```python
from build123d import *

# Parameters (mm, degrees)
SKETCH_1_W          = 20
SKETCH_1_H          = 19
SKETCH_1_R          = 3
EXTRUDE_1_DEPTH     = 18
SKETCH_1_H_2        = 20
EXTRUDE_1_2_DEPTH   = 18
SKETCH_2_W          = 20
SKETCH_2_H          = 109
SKETCH_2_R          = 3
EXTRUDE_2_DEPTH     = 4
EXTRUDE_3_DEPTH     = 6
SKETCH_4_R          = 0.9
CUT_EXTRUDE_1_DEPTH = 788.391009845
SKETCH_5_R          = 3
EXTRUDE_4_DEPTH     = 13
CHAMFER_1_SIZE      = 2
SKETCH_6_W          = 3.5
SKETCH_6_H          = 12.5
EXTRUDE_5_DEPTH     = 5
FILLET_1_R          = 4
CHAMFER_2_SIZE      = 2


with BuildPart() as part:
    # Sketch 1 → Extrude 1 (new body)
    with BuildSketch(Plane(origin=(0, 0, 241.9894311), x_dir=(-1, 0, 0), z_dir=(0, 0, -1))):
        with Locations((770.850538245, -0.64131648)):
            Rectangle(SKETCH_1_W, SKETCH_1_H)
        with Locations(Location((770.850538245, -1.14131648, 0), (0, 0, 90))):
            Circle(SKETCH_1_R, mode=Mode.SUBTRACT)
    extrude(amount=EXTRUDE_1_DEPTH)



with BuildPart() as body_2:
    # Sketch 1 → Extrude 1 2 (new body)
    with BuildSketch(Plane(origin=(0, 0, 241.9894311), x_dir=(-1, 0, 0), z_dir=(0, 0, -1))):
        with Locations((770.850538245, 88.85868352)):
            Rectangle(SKETCH_1_W, SKETCH_1_H_2)
        with Locations(Location((770.850538245, 88.85868352, 0), (0, 0, 90))):
            Circle(SKETCH_1_R, mode=Mode.SUBTRACT)
    extrude(amount=EXTRUDE_1_2_DEPTH)


with BuildPart() as part_1:
    add(part.part)

    add(body_2.part)  # Extrude 2 merges body 2
    # Sketch 2 → Extrude 2 (add)
    with BuildSketch(Plane(origin=(0, 0, 223.9894311), x_dir=(-1, 0, 0), z_dir=(0, 0, -1))):
        with Locations((770.850538245, 44.35868352)):
            Rectangle(SKETCH_2_W, SKETCH_2_H)
        with Locations(Location((770.850538245, 88.85868352, 0), (0, 0, 90))):
            Circle(SKETCH_2_R, mode=Mode.SUBTRACT)
        with Locations(Location((770.850538245, -1.14131648, 0), (0, 0, 90))):
            Circle(SKETCH_2_R, mode=Mode.SUBTRACT)
    extrude(amount=EXTRUDE_2_DEPTH)

    # Sketch 3 → Extrude 3 (add)
    with BuildSketch(Plane(origin=(0, 0, 219.9894311), x_dir=(-1, 0, 0), z_dir=(0, 0, -1))):
        Polygon((780.850538245, 59.85868352), (780.850538245, 51.85868352), (777.850538245, 51.85868352), (777.850538245, 48.60868352), (769.850538245, 48.60868352), (769.850538245, 61.10868352), (777.850538245, 61.10868352), (777.850538245, 59.85868352), align=None)
    extrude(amount=EXTRUDE_3_DEPTH)

    # Sketch 4 → Cut-Extrude 1 (cut, through all)
    with BuildSketch(Plane(origin=(0, 0, 219.9894311), x_dir=(-1, 0, 0), z_dir=(0, 0, -1))):
        with Locations(Location((775.850538245, 50.85868352, 0), (0, 0, 90))):
            Circle(SKETCH_4_R)
        with Locations(Location((775.850538245, 58.85868352, 0), (0, 0, 90))):
            Circle(SKETCH_4_R)
    extrude(amount=CUT_EXTRUDE_1_DEPTH, mode=Mode.SUBTRACT)

    # Sketch 5 → Extrude 4 (add)
    # profile 1 of 2: a face of its own
    with BuildSketch(Plane(origin=(0, 0, 219.9894311), x_dir=(-1, 0, 0), z_dir=(0, 0, -1))):
        Polygon((760.850538245, -10.14131648), (780.850538245, -10.14131648), (780.850538245, 51.85868352), (777.850538245, 51.85868352), (777.850538245, 48.60868352), (760.850538245, 48.60868352), align=None)
        with Locations(Location((770.850538245, -1.14131648, 0), (0, 0, 90))):
            Circle(SKETCH_5_R, mode=Mode.SUBTRACT)
    # profile 2 of 2: a face of its own
    with BuildSketch(Plane(origin=(0, 0, 219.9894311), x_dir=(-1, 0, 0), z_dir=(0, 0, -1))):
        Polygon((777.850538245, 61.10868352), (777.850538245, 59.85868352), (780.850538245, 59.85868352), (780.850538245, 98.85868352), (760.850538245, 98.85868352), (760.850538245, 61.10868352), align=None)
        with Locations(Location((770.850538245, 88.85868352, 0), (0, 0, 90))):
            Circle(SKETCH_5_R, mode=Mode.SUBTRACT)
    extrude(amount=EXTRUDE_4_DEPTH)

    # Chamfer 1
    chamfer_1_edges = [part_1.edges().sort_by_distance(p)[0] for p in [
        (-780.850538245, 59.85868352, 210.4894311),
        (-780.850538245, 55.85868352, 213.9894311),
        (-780.850538245, 51.85868352, 210.4894311),
    ]]
    chamfer(chamfer_1_edges, length=CHAMFER_1_SIZE)

    # Sketch 6 → Extrude 5 (add)
    with BuildSketch(Plane(origin=(0, 0, 206.9894311), x_dir=(-1, 0, 0), z_dir=(0, 0, -1))):
        with Locations((762.600538245, 54.85868352)):
            Rectangle(SKETCH_6_W, SKETCH_6_H)
    extrude(amount=-EXTRUDE_5_DEPTH)

    # Fillet 1
    fillet_1_edges = [part_1.edges().sort_by_distance(p)[0] for p in [
        (-780.850538245, 98.85868352, 224.4894311),
        (-780.850538245, 78.85868352, 232.9894311),
        (-780.850538245, 8.85868352, 232.9894311),
        (-780.850538245, -10.14131648, 224.4894311),
    ]]
    fillet(fillet_1_edges, radius=FILLET_1_R)

    # Chamfer 2
    chamfer_2_edges = [part_1.edges().sort_by_distance(p)[0] for p in [
        (-760.850538245, 98.85868352, 224.4894311),
        (-760.850538245, -10.14131648, 224.4894311),
    ]]
    chamfer(chamfer_2_edges, length=CHAMFER_2_SIZE)


solid = part_1.part
```
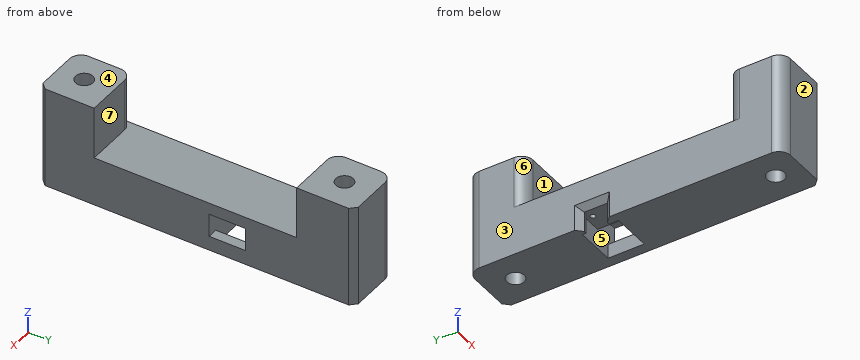
Build history of the part. All positions in model axes, mm. Face numbers are marked on the shaded views. A direction names the side the tool comes from. Coordinates: 2 decimals unless noted, no trailing zeros. Order: outer loops, then holes, each group sorted by start corner. A loop starts at its lowest first (then second) coordinate and runs counter-clockwise, first axis right, second up.
Item 1: Drop flat-ended pins along their axis: pin 1 Ø2 at (x, y) = (-776, 50.5) entering from -Z; pin 2 Ø1.1 at (x, z) = (-778.5, 210.5) entering from +Y; pin 3 Ø10 at (x, y) = (-772.5, 52) entering from +Z; pin 4 Ø5 at (x, y) = (-770.85, 88.86) entering from -Z. Give the stop position or say it passes through.
Filled in:
pin 1: stops at z = 213.99
pin 2: stops at y = 98.7
pin 3: stops at z = 223.99
pin 4: passes through
Item 2: Saw through at D-D on z = 215. List the corners of the cut face in (x, y), then the cut area to 3 significant figures.
Filled in:
outline: (-780.85, -6.14) arc R4 ccw to (-776.85, -10.14) - (-762.85, -10.14) - (-760.85, -8.14) - (-760.85, 48.61) - (-769.85, 48.61) - (-769.85, 61.11) - (-760.85, 61.11) - (-760.85, 96.86) - (-762.85, 98.86) - (-776.85, 98.86) arc R4 ccw to (-780.85, 94.86) - (-780.85, 61.86) - (-779.86, 60.87) - (-779.86, 50.85) - (-780.85, 49.86) - close; hole circle Ø1.8 at (-775.85, 50.86); hole circle Ø1.8 at (-775.85, 58.86); hole circle Ø6 at (-770.85, -1.14); hole circle Ø6 at (-770.85, 88.86)
area: 1,980 mm2
Item 3: Saw through at A-A on y = 55. List the corners of the cut face in (x, z), then the cut area to 4 significant figures.
Filled in:
outline: (-780.85, 215.99) - (-778.85, 213.99) - (-769.85, 213.99) - (-769.85, 219.99) - (-760.85, 219.99) - (-760.85, 223.99) - (-780.85, 223.99) - close; (-764.35, 206.99) - (-760.85, 206.99) - (-760.85, 211.99) - (-764.35, 211.99) - close
area: 161.5 mm2
Item 4: Mould opens along Y. For the marked faces 1, 2 and 3 say: released by +Y, released by -Y, zero draft, split by the parting line, or undercut.
Filled in:
face 1: undercut
face 2: released by -Y
face 3: zero draft
Item 5: Saw through at C-C on x = -772. List the corners of the cut face in (y, z), then the cut area to 3 significant figures.
Filled in:
outline: (-10.14, 206.99) - (-3.91, 206.99) - (-3.91, 241.99) - (-10.14, 241.99) - close; (1.63, 206.99) - (48.61, 206.99) - (48.61, 213.99) - (61.11, 213.99) - (61.11, 206.99) - (86.09, 206.99) - (86.09, 241.99) - (78.86, 241.99) - (78.86, 223.99) - (8.86, 223.99) - (8.86, 241.99) - (1.63, 241.99) - close; (91.63, 206.99) - (98.86, 206.99) - (98.86, 241.99) - (91.63, 241.99) - close
area: 2,080 mm2
Item 6: Tool access for the marked faces 4, 5, 6 and 7: list every direction of +Z, -Z, +X, -X, +Y, -Y with a clear straight run to the whole face (end or side of a thin tool).
Filled in:
face 4: +Z, +X, -X, +Y, -Y
face 5: none
face 6: +Z, -X
face 7: +Z, +X, -X
Item 7: Drill centre lines: L1, parallel to Y at x = -770.75, z = 237.5; L2, parallel to Y at x = -773.5, z = 235; L3, parallel to Y at x = -766, z = 225.5. Where is each one in solid material? Low to high.
Filled in:
L1: y = -10.14 to -4.14, 1.86 to 8.86, 78.86 to 85.86, 91.86 to 98.86
L2: y = -10.14 to -2.55, 0.27 to 8.86, 78.86 to 87.45, 90.27 to 98.86
L3: y = -10.14 to 8.86, 78.86 to 98.86
Item 8: Saw through at B-B on z = 239. List the corners of the cut face in (x, y), then the cut area to 3 significant figures.
Filled in:
outline: (-780.85, -6.14) arc R4 ccw to (-776.85, -10.14) - (-762.85, -10.14) - (-760.85, -8.14) - (-760.85, 8.86) - (-776.85, 8.86) arc R4 ccw to (-780.85, 4.86) - close; (-780.85, 82.86) arc R4 ccw to (-776.85, 78.86) - (-760.85, 78.86) - (-760.85, 96.86) - (-762.85, 98.86) - (-776.85, 98.86) arc R4 ccw to (-780.85, 94.86) - close; hole circle Ø6 at (-770.85, -1.14); hole circle Ø6 at (-770.85, 88.86)
area: 706 mm2
